Design review of the part built by this model. Coordinates are the model's own, in mm. Coordinates: 2 decimals unless noted, no trailing zeros. Write each loop counter-clockwise with the first axis right and the second up, starting at its lowest first coordinate (ties: lowest second). Pieces come first, ordered by that corner, then holes. Notation, with made-up numbers: M 87,22.5 L 123,22.5 A19 ccw 123,52.5 Z; hole C -27.75,3 d10. An arc over 180 degrees is marked long. Write item = value, one per line.
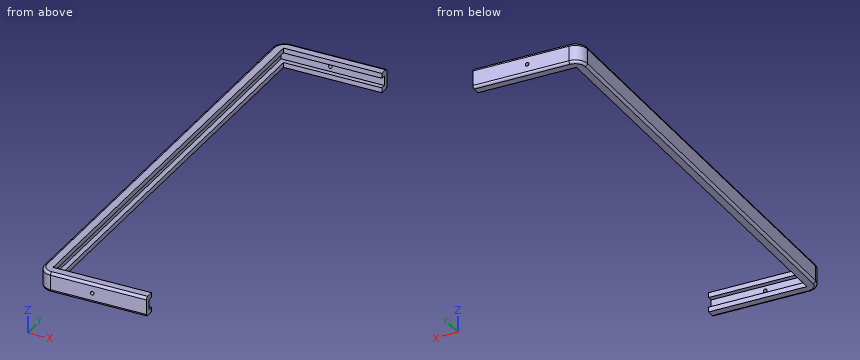
```python
from build123d import *

# Parameters (mm, degrees)
F0_W     = 1880
F0_H     = 80
F1_DEPTH = 440
F2_W     = 1800
F2_H     = 80
F3_DEPTH = 400
F4_W     = 400
F4_H     = 40
F5_DEPTH = 20
F6_W     = 400
F6_H     = 40
F7_DEPTH = 20
F8_W     = 1840
F8_H     = 40
F9_DEPTH = 20
F11_D    = 15
F12_R    = 50
F13_R    = 50
F14_R    = 10


with BuildPart() as f1:
    # F0 (on Right) → F1 (new body)
    with BuildSketch(Plane.YZ):
        with Locations((818.311098, -14.702874)):
            Rectangle(F0_W, F0_H)
    extrude(amount=F1_DEPTH)

    # F2 (on face) → F3 (cut)
    with BuildSketch(Plane.YZ.offset(440)):
        with Locations((818.311098, -14.702874)):
            Rectangle(F2_W, F2_H)
    extrude(amount=-F3_DEPTH, mode=Mode.SUBTRACT)

    # F4 (on face) → F5 (cut)
    with BuildSketch(Plane.XZ.offset(-1718.311098)):
        with Locations((240, -14.702874)):
            Rectangle(F4_W, F4_H)
    extrude(amount=-F5_DEPTH, mode=Mode.SUBTRACT)

    # F6 (on face) → F7 (cut)
    with BuildSketch(Plane(origin=(0, -81.688902, 0), x_dir=(-1, 0, 0), z_dir=(0, 1, 0))):
        with Locations((-240, -14.702874)):
            Rectangle(F6_W, F6_H)
    extrude(amount=-F7_DEPTH, mode=Mode.SUBTRACT)

    # F8 (on face) → F9 (cut)
    with BuildSketch(Plane.YZ.offset(40)):
        with Locations((818.311098, -14.702874)):
            Rectangle(F8_W, F8_H)
    extrude(amount=-F9_DEPTH, mode=Mode.SUBTRACT)

    # F11 (through all)
    with Locations(Plane(origin=(0, 1758.311098, 0), x_dir=(-1, 0, 0), z_dir=(0, 1, 0))):
        with Locations((-220, -14.702874)):
            Hole(F11_D / 2)

    # F12
    f12_edges = [f1.edges().sort_by_distance(p)[0] for p in [
        (0, 1758.311098, -14.702874),
    ]]
    fillet(f12_edges, radius=F12_R)

    # F13
    f13_edges = [f1.edges().sort_by_distance(p)[0] for p in [
        (0, -121.688902, -14.702874),
    ]]
    fillet(f13_edges, radius=F13_R)

    # F14
    f14_edges = [f1.edges().sort_by_distance(p)[0] for p in [
        (0, 818.311098, -54.702874),
        (0, 818.311098, 25.297126),
    ]]
    fillet(f14_edges, radius=F14_R)


solid = f1.part
```
Q1. Consider section A-A, the plane x = 161. State the section outline as (y, z) points, and give its area (3 significant figures).
Check result:
outline = M -121.69,-44.7 A10 ccw -111.69,-54.7 L -81.69,-54.7 L -81.69,-34.7 L -101.69,-34.7 L -101.69,5.3 L -81.69,5.3 L -81.69,25.3 L -111.69,25.3 A10 ccw -121.69,15.3 Z; M 1718.31,-54.7 L 1748.31,-54.7 A10 ccw 1758.31,-44.7 L 1758.31,15.3 A10 ccw 1748.31,25.3 L 1718.31,25.3 L 1718.31,5.3 L 1738.31,5.3 L 1738.31,-34.7 L 1718.31,-34.7 Z
area = 4,710 mm²
Q2. For P1, Ø16, axis at y = 798.5, z = -48.5, coming from the +X side; P2, Ø9, axis at x = 220, z = -14.7, coming from the +Y side; P3, Ø12, axis at y = 1050.5, z = -17.5, coming from the +X side, all flat-tipped, find the tip position at first contact; note any pin that passes through.
Check result:
P1 = 40
P2 = through
P3 = 20
Q3. Wall thickness on line 1 (Z direction, x = 220, y = -108); line 2 (Y direction, x = 345, z = 16); line 3 (Y direction, x = 276, z = -1.5): over which ranges is each line inside the solid? List them lowest first.
Check result:
line_1 = -54.7 to -22.2, -7.2 to 25.3
line_2 = -121.66 to -81.69, 1718.31 to 1758.29
line_3 = -121.69 to -101.69, 1738.31 to 1758.31
Q4. Consider section B-B, the plane y = 182. State the section outline as (x, z) points.
Check result:
outline = M 0,-44.7 A10 ccw 10,-54.7 L 40,-54.7 L 40,-34.7 L 20,-34.7 L 20,5.3 L 40,5.3 L 40,25.3 L 10,25.3 A10 ccw 0,15.3 Z
